The listing builds one solid part. Answer for the finished solid, in the listing's coordinates (mm). Coordinates: 2 decimals unless noted, no trailing zeros. Answer in a Markdown table with one row per item.
Autodesk Inventor part; units mm, degrees
ref_plane "Arbeitsebene1" through (0, 800, 0) normal (0, 1, 0) x (-1, 0, 0)
ref_plane "YZ Plane" through (0, 0, 0) normal (1, 0, 0) x (0, 1, 0)
ref_plane "XY Plane" through (0, 0, 0) normal (0, 0, 1) x (1, 0, 0)
sketch "ground" plane through (0, 0, 0) normal (0, 1, 0) x (-1, 0, 0)
  line L0 (483.3377, 0) -> (445.9963, 94.5527) construction
  line L1 (445.9963, 94.5527) -> (-16.6623, 0) construction
  spline S0 degree 2 poles (483.3377, 0) (445.9963, 94.5527) (-16.6623, 0) knots 1 1 1 2 2 2
  line L2 (483.3377, 0) -> (-16.6623, 0)
  point P0 (0, 0)
  dimension "d0" = 500
  dimension "d21" = 100
  dimension "d22" = 68.45
ref_plane "Arbeitsebene1" through (0, 800, 0) normal (0, 1, 0) x (-1, 0, 0)
sketch "Skizze3" plane through (0, 800, 0) normal (0, 1, 0) x (-1, 0, 0)
  line L0 (483.3697, 0) -> (460.9649, 56.7316) construction
  line L1 (460.9649, 56.7316) -> (183.3697, 0) construction
  spline S0 degree 2 poles (483.3697, 0) (460.9649, 56.7316) (183.3697, 0) knots 1 1 1 2 2 2
  line L2 (483.3697, 0) -> (183.3697, 0)
  point P0 (0, 0)
  dimension "d27" = 300
  dimension "d28" = 100
  dimension "d29" = 68.45
sketch "Skizze5" plane through (0, 800, 0) normal (0, 1, 0) x (-1, 0, 0)
  circle A0 centre (434.5806, 0) radius 12.3812
  point P0 (0, 0)
loft "Erhebung2" add profiles "ground", "Skizze3"
mirror "Spiegeln2" about plane through (16.6623, 0, 0) normal (0, 0, -1) of "Erhebung2"
hole "Bohrung1" at (-434.5806, 800, 0) direction (0, -1, 0) diameter 25 end through all
properties part number "mb_sail"
Item 1: Determine the mould class of faces 1 (the face through (-272, 0, -7)), 2 (the face through (-446.974, 394.4, -1.627)) for opening direction Z: +Z half, -Z half, draft (parallel to the pull), parting line (faces both ways), or undercut.
Findings below:
| item | result |
|---|---|
| face 1 | draft |
| face 2 | undercut |
Item 2: Flat-ended cylindrical pins translate along their axes: pin 1 Ø1.5 at (x, y) = (-252, 255) entering from +Z; pin 2 Ø4 at (x, y) = (-87, 404) entering from -Z; pin 3 Ø2 at (x, y) = (-341.5, 697) entering from -Z. Find the tip coordinate at first contact, or state that the pin passes through.
Findings below:
| item | result |
|---|---|
| pin 1 | stops at z = 34.29 |
| pin 2 | stops at z = -0.96 |
| pin 3 | stops at z = -28.71 |
Item 3: Find the intervals of material crossed by probe 1 along Z at (x, y) = (-297, 697); probe 2 along Z at (x, y) = (-173.5, 268), in increasing order.
Findings below:
| item | result |
|---|---|
| probe 1 | z = -23.88 to 23.88 |
| probe 2 | z = -22.72 to 22.72 |
